```python
from build123d import *

# Parameters (mm, degrees)
BOSS_EXTRUDE1_DEPTH  = 10
SKETCH6_R            = 4
BOSS_EXTRUDE3_DEPTH  = 18
FILLET2_R            = 1
FILLET2_OF_MIRROR1_R = 1
SKETCH7_W            = 18
SKETCH7_H            = 5
BOSS_EXTRUDE4_DEPTH  = 8.5


with BuildPart() as part:
    # Sketch2 → Boss-Extrude1 (new body)
    with BuildSketch(Plane.XY):
        Polygon((0, 58.642667291), (0, 38.642667291), (15, 38.642667291), (19.305964995, 31.988891988), (19.305964995, -34.929478391), (0, -34.929478391), (0, -49.929478391), (15, -49.929478391), (15, -96.857332709), (0, -96.857332709), (0, -111.857332709), (112.395493867, -111.857332709), (125.33841664, -131.857332709), (150.33841664, -131.857332709), (150.33841664, -111.857332709), (135.33841664, -111.857332709), (15, 58.642667291), align=None)
        Polygon((27, -49.929478391), (72.31912207, -49.929478391), (102.688301787, -96.857332709), (27, -96.857332709), align=None, mode=Mode.SUBTRACT)
        Polygon((31.305964995, -34.929478391), (31.305964995, 13.445939657), (62.61192999, -34.929478391), align=None, mode=Mode.SUBTRACT)
    boss_extrude1 = extrude(amount=BOSS_EXTRUDE1_DEPTH)

    # Sketch6 → Boss-Extrude3 (add)
    with BuildSketch(Plane(origin=(150.33841664, 0, 0), x_dir=(0, 0, -1), z_dir=(1, 0, 0))):
        with Locations(Location((-5, -121.857332709, 0), (0, 0, 90))):
            Circle(SKETCH6_R)
    boss_extrude3 = extrude(amount=BOSS_EXTRUDE3_DEPTH)

    # Fillet2
    fillet2_edges = [part.edges().sort_by_distance(p)[0] for p in [
        (150.33841664, -125.857332709, 5),
    ]]
    fillet(fillet2_edges, radius=FILLET2_R - 0.0001)  # a hair under: the kernel refuses the full size

    # Mirror1: Boss-Extrude1, Boss-Extrude3 across plane
    add(boss_extrude1.mirror(Plane(origin=(0, 0, 10), x_dir=(0, 0, 1), z_dir=(1, 0, 0))))
    add(boss_extrude3.mirror(Plane(origin=(0, 0, 10), x_dir=(0, 0, 1), z_dir=(1, 0, 0))))

    # Fillet2 of Mirror1
    fillet2_of_mirror1_edges = [part.edges().sort_by_distance(p)[0] for p in [
        (-150.33841664, -125.857332709, 5),
    ]]
    fillet(fillet2_of_mirror1_edges, radius=FILLET2_OF_MIRROR1_R - 0.0001)  # a hair under: the kernel refuses the full size

    # Sketch7 → Boss-Extrude4 (add)
    with BuildSketch(Plane(origin=(0, 58.642667291, 0), x_dir=(1, 0, 0), z_dir=(0, 1, 0))):
        with Locations((0, -5)):
            Rectangle(SKETCH7_W, SKETCH7_H)
    extrude(amount=BOSS_EXTRUDE4_DEPTH)


solid = part.part
```
Here's how the part is built. I have some questions about the finished solid (model axes, mm). A direction names the side the tool comes from. Round coordinates to 2 decimals unless told otherwise and drop trailing zeros. Write each loop counter-clockwise with the first axis right and the second up, starting at its lowest first coordinate (ties: lowest second). Pieces come first, ordered by that corner, then holes.
Q1. Will these pins go through, and if not, where does the flat tip stop? P1, Ø4, axis at x = -48, z = 4.5, coming from the -Y side; P2, Ø4, axis at y = -17, z = 8.5, coming from the -X side; P3, Ø7, axis at x = 2, y = 63, coming from the +Z side.
Q2. If we section it at B-B on z = 5: Give the number of separate pieces and of enclosed holes in the cut face, plus the area to 3 significant figures.
Q3. If we section it at D-D on x = 107.5: Write out the boundary of the cut face in (y, z), plus the area to 3 significant figures.
Q4. If we section it at A-A on y = 0: Write out the boundary of the cut face in (x, z), plus the area to 3 significant figures.
Q5. If we section it at C-C on y = -91.5: Write out the boundary of the cut face in (x, z).
Q6. Which directions (+Z, -Z, +X, -X, +Y, -Y) give clear straight access to the entire face, cutting with the end or side of a thin tool? Please do faces 1 (the flat face through (-31.306, -11, 5)), 2 (the flat face through (143, -111.857, 5)), 3 (the flat face through (12, -43, 10)), 4 (the flat face through (2, -111.857, 5)), 5 (the flat face through (12, -43, 0)).
Q7. If we mould it in two halves opening along X, with no side actions, what happens to faces 6 (the flat face through (-76.01, -27.8, 4.93)), 7 (the flat face through (46.74, -10.4, 4.93)), 8 (the flat face through (150.338, -126.4, 1.6)), 9 (the cylindrical face through (-159.72, -118.16, 3.47))? For each: +X half, -X half, draft (parallel to the pull), parting line (faces both ways), or undercut.
Q8. Please list where these lines run through material, in increasing order: probe 1 along Y at (x, z) = (-40, 4.75); probe 2 along X at (y, z) = (-51, 6.25); probe 3 along Y at (x, z) = (-14, 4.75).
Answer below:
1. P1: stops at y = -111.86
1. P2: stops at x = -69.8
1. P3: stops at z = 7.5
2. separate pieces: 1
2. enclosed holes: 6
2. area: 15,900 mm2
3. outline: (-111.86, 0) - (-72.41, 0) - (-72.41, 10) - (-111.86, 10) - close
3. area: 394 mm2
4. outline: (-56.39, 0) - (-40.01, 0) - (-40.01, 10) - (-56.39, 10) - close; (-31.31, 0) - (-19.31, 0) - (-19.31, 10) - (-31.31, 10) - close; (19.31, 0) - (31.31, 0) - (31.31, 10) - (19.31, 10) - close; (40.01, 0) - (56.39, 0) - (56.39, 10) - (40.01, 10) - close
4. area: 568 mm2
5. outline: (-120.97, 0) - (-99.22, 0) - (-99.22, 10) - (-120.97, 10) - close; (-27, 0) - (-15, 0) - (-15, 10) - (-27, 10) - close; (15, 0) - (27, 0) - (27, 10) - (15, 10) - close; (99.22, 0) - (120.97, 0) - (120.97, 10) - (99.22, 10) - close
6. face 1: +Z, -Z
6. face 2: +Z, -Z, +X, +Y
6. face 3: +Z, +X, -X, +Y, -Y
6. face 4: +Z, -Z, -Y
6. face 5: -Z, +X, -X, +Y, -Y
7. face 6: -X half
7. face 7: undercut
7. face 8: +X half
7. face 9: draft
8. probe 1: y = -111.86 to -96.86, -49.93 to -34.93, 0.01 to 23.22
8. probe 2: x = -92.39 to -73.01, -27 to -15, 15 to 27, 73.01 to 92.39
8. probe 3: y = -111.86 to -96.86, -49.93 to -34.93, 38.64 to 58.64
